```python
from build123d import *

# Parameters (mm, degrees)
F0_R     = 5.25
F1_DEPTH = 10
F2_R     = 5
F3_R     = 5


with BuildPart() as f1:
    # F0 (on Front) → F1 (new body)
    with BuildSketch(Plane.XZ):
        Polygon((-250, 62.760484), (-450, 62.760484), (-450, -237.239516), (0, -237.239516), (450, -237.239516), (450, 62.760484), (250, 62.760484), (125, 237.760484), (125, 362.760484), (-125, 362.760484), (-125, 237.760484), align=None)
        with Locations((-416.203916, -217.239516)):
            Circle(F0_R, mode=Mode.SUBTRACT)
        with Locations((-396.203916, -217.239516)):
            Circle(F0_R, mode=Mode.SUBTRACT)
        with BuildLine():
            Line((-357.815236, -90.926083), (-77.815236, -90.926083))
            ThreePointArc((-77.815236, -90.926083), (-55.315236, -113.426083), (-77.815236, -135.926083))
            Line((-77.815236, -135.926083), (-357.815236, -135.926083))
            ThreePointArc((-357.815236, -135.926083), (-380.315236, -113.426083), (-357.815236, -90.926083))
        make_face(mode=Mode.SUBTRACT)
        Polygon((-292.343991, -60), (-292.343991, 0), (-230.370536, 0), (-117.343991, 165), (-67.343991, 165), (-67.343991, 0), (-67.343991, -60), align=None, mode=Mode.SUBTRACT)
        with BuildLine():
            ThreePointArc((77.815236, -135.926083), (55.315236, -113.426083), (77.815236, -90.926083))
            Line((77.815236, -90.926083), (357.815236, -90.926083))
            ThreePointArc((357.815236, -90.926083), (380.315236, -113.426083), (357.815236, -135.926083))
            Line((357.815236, -135.926083), (77.815236, -135.926083))
        make_face(mode=Mode.SUBTRACT)
        with Locations((416.841447, -217.239516)):
            Circle(F0_R, mode=Mode.SUBTRACT)
        with Locations((436.841447, -217.239516)):
            Circle(F0_R, mode=Mode.SUBTRACT)
        Polygon((67.343991, 0), (67.343991, 165), (117.343991, 165), (230.370536, 0), (292.343991, 0), (292.343991, -60), (67.343991, -60), align=None, mode=Mode.SUBTRACT)
        with Locations((-86.261913, 342.760484)):
            Circle(F0_R, mode=Mode.SUBTRACT)
        with BuildLine():
            Line((-10.5, 0), (-10.5, 235.897347))
            ThreePointArc((-10.5, 235.897347), (0, 246.397347), (10.5, 235.897347))
            Line((10.5, 235.897347), (10.5, 0))
            Line((10.5, 0), (10.5, -70.725352))
            ThreePointArc((10.5, -70.725352), (0, -81.225352), (-10.5, -70.725352))
            Line((-10.5, -70.725352), (-10.5, 0))
        make_face(mode=Mode.SUBTRACT)
        with Locations((86.048543, 342.760484)):
            Circle(F0_R, mode=Mode.SUBTRACT)
    extrude(amount=F1_DEPTH)

    # F2
    f2_edges = [f1.edges().sort_by_distance(p)[0] for p in [
        (-230.370536, -5, 0),
        (230.370536, -5, 0),
    ]]
    fillet(f2_edges, radius=F2_R)

    # F3
    f3_edges = [f1.edges().sort_by_distance(p)[0] for p in [
        (-450, -5, 62.760484),
        (-125, -5, 362.760484),
        (125, -5, 362.760484),
        (450, -5, 62.760484),
    ]]
    fillet(f3_edges, radius=F3_R)


solid = f1.part
```
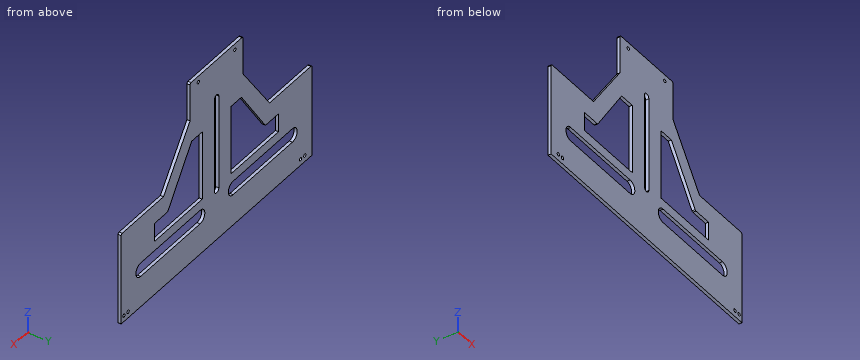
Model file for the job. Use its own axes, mm. Give positions to 0.01 mm unless a question says otherwise; leave off trailing zeros. Loops run counter-clockwise (first coordinate to the right, second up) from the corner with the lowest first, then second, coordinate; pieces in that order, holes last. Notation, with made-up numbers: (28.5, 6.25) - (61.5, 6.25) arc R7 ccw to (61.5, 11.25) - close; hole circle Ø11 at (-19, 14). An arc over 180 degrees is marked (long way). One line per item, written item: value. Start each with the question number.
1. Slice it at B-B (z = 91). List the corners of the cut face in (x, y).
2. Probe L1, parallel to X at y = -8, z = -51; L2, parallel to Z at x = 342, y = -1.25; L3, parallel to Z at x = -147, y = -0.5. List the from-to ranges inside material, lowest first. Write a range as from..to.
3. Pin check, flat tip, straight feed: pin 1 (5 mm diameter, centred on x = 388, y = -6.5, fed in from +Z). Stop position of the tip, or through.
4. Slice it at A-A (x = 314). List the corners of the cut face in (y, z), plus the area to 3 significant figures.
5. Slice it at D-D (x = 0). List the corners of the cut face in (y, z), plus the area to 3 significant figures.
6. Slice it at C-C (x = -262.5). List the corners of the cut face in (y, z).
Solution:
1. outline: (-229.83, -10) - (-168.03, -10) - (-168.03, 0) - (-229.83, 0) - close; (-67.34, -10) - (-10.5, -10) - (-10.5, 0) - (-67.34, 0) - close; (10.5, -10) - (67.34, -10) - (67.34, 0) - (10.5, 0) - close; (168.03, -10) - (229.83, -10) - (229.83, 0) - (168.03, 0) - close
2. L1: x = -450..-292.34, -67.34..-10.5, 10.5..67.34, 292.34..450
2. L2: z = -237.24..-135.93, -90.93..62.76
2. L3: z = -237.24..-135.93, -90.93..-60, 121.71..206.96
3. pin 1: stops at z = 62.76
4. outline: (-10, -237.24) - (0, -237.24) - (0, -135.93) - (-10, -135.93) - close; (-10, -90.93) - (0, -90.93) - (0, 62.76) - (-10, 62.76) - close
4. area: 2,550 mm^2
5. outline: (-10, -237.24) - (0, -237.24) - (0, -81.23) - (-10, -81.23) - close; (-10, 246.4) - (0, 246.4) - (0, 362.76) - (-10, 362.76) - close
5. area: 2,720 mm^2
6. outline: (-10, -237.24) - (0, -237.24) - (0, -135.93) - (-10, -135.93) - close; (-10, -90.93) - (0, -90.93) - (0, -60) - (-10, -60) - close; (-10, 0) - (0, 0) - (0, 62.76) - (-10, 62.76) - close
